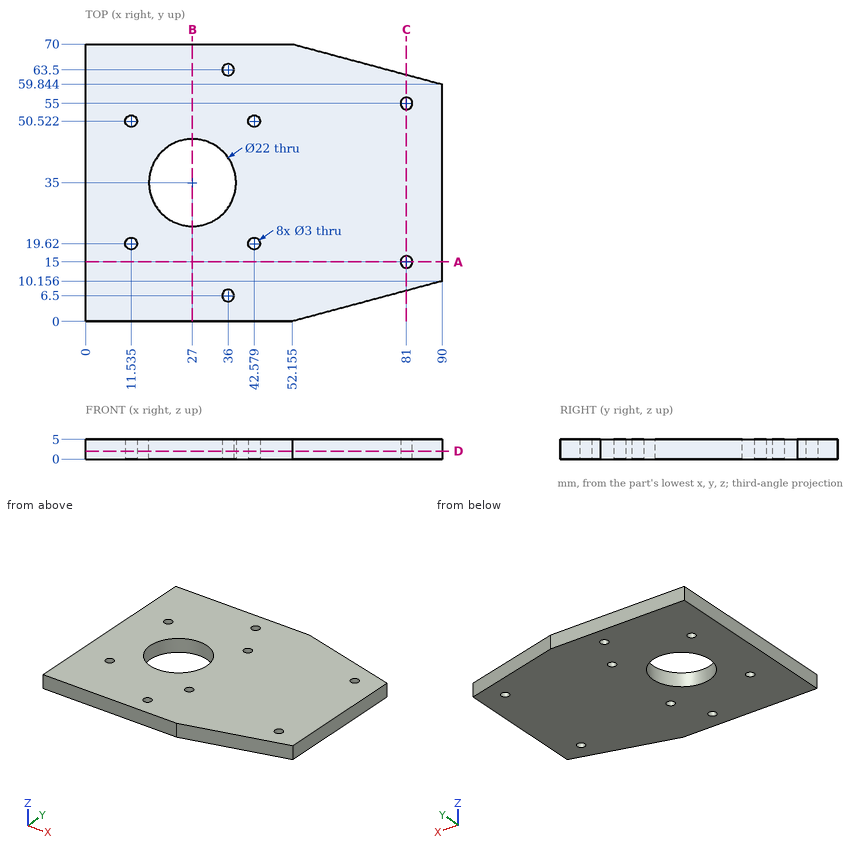
Verification items for this drawing (mm, ordinates from the low corner). Round coordinates to 2 decimals unless told otherwise and drop trailing zeros. Loops run counter-clockwise (first coordinate to the right, second up) from the corner with the lowest first, then second, coordinate; pieces in that order, holes last. Notation, with made-up numbers: (14, 65.25) - (64, 65.25) arc R24 ccw to (64, 86.25) - close; hole circle Ø8 at (-5.5, 63.25). An arc over 180 degrees is marked (long way). Write item = value, one per line.
Q1. Sectioned sample at C-C on x = 81. Record the boundary of the cut face in (y, z).
Here are the results:
outline = (7.74, 0) - (13.5, 0) - (13.5, 5) - (7.74, 5) - close; (16.5, 0) - (53.5, 0) - (53.5, 5) - (16.5, 5) - close; (56.5, 0) - (62.26, 0) - (62.26, 5) - (56.5, 5) - close
Q2. Sectioned sample at A-A on y = 15. Record the boundary of the cut face in (x, z).
Here are the results:
outline = (0, 0) - (79.5, 0) - (79.5, 5) - (0, 5) - close; (82.5, 0) - (90, 0) - (90, 5) - (82.5, 5) - close
Q3. Sectioned sample at B-B on x = 27. Record the boundary of the cut face in (y, z), plus the area to 3 significant figures.
Here are the results:
outline = (0, 0) - (24, 0) - (24, 5) - (0, 5) - close; (46, 0) - (70, 0) - (70, 5) - (46, 5) - close
area = 240 mm^2
Q4. Depth check by flat-ended pin: pin 1 (4 mm diameter, centred on x = 81, y = 15, fed in from -Z); pin 2 (2.5 mm diameter, centred on x = 36, y = 63.5, fed in from -Z). Enter the tip coordinate at first touch or a pass-through.
Here are the results:
pin_1 = 0
pin_2 = through
Q5. Material ranges on L1, parallel to Y at x = 36, z = 3.8 (1 decimal); L2, parallel to Y at x = 81, z = 1.1; L3, parallel to X at y = 19, z = 3.25 (1 decimal), recorded low to high.
Here are the results:
L1 = 0 to 5, 8 to 28.7, 41.3 to 62, 65 to 70
L2 = 7.74 to 13.5, 16.5 to 53.5, 56.5 to 62.26
L3 = 0 to 10.2, 12.9 to 41.2, 43.9 to 90
Q6. Sectioned sample at D-D on z = 2.05. State how many separate pieces and enclosed holes the cut face has, plus the area to 3 significant figures.
Here are the results:
separate_pieces = 1
enclosed_holes = 9
area = 5,480 mm^2
